from build123d import *

# Parameters (mm, degrees)
SKETCH1_R                  = 10
BOSS_EXTRUDE1_DEPTH        = 30
SKETCH2_R                  = 5.005
CUT_EXTRUDE1_DEPTH         = 20
CUT_EXTRUDE2_DEPTH         = 10
SKETCH4_R                  = 8
CUT_EXTRUDE3_DEPTH         = 4.01
M2X0_4_TAPPED_HOLE1_REACH  = 39.417
M2X0_4_TAPPED_HOLE1_BORE_R = 0.8
M2X0_4_TAPPED_HOLE2_D      = 1.6
M2X0_4_TAPPED_HOLE3_D      = 1.6
M2X0_4_TAPPED_HOLE4_REACH  = 39.417
M2X0_4_TAPPED_HOLE4_BORE_R = 0.8


with BuildPart() as part:
    # Sketch1 → Boss-Extrude1 (new body)
    with BuildSketch(Plane(origin=(0, 0, 0), x_dir=(0, 0, -1), z_dir=(1, 0, 0))):
        Circle(SKETCH1_R)
    extrude(amount=BOSS_EXTRUDE1_DEPTH)

    # Sketch2 → Cut-Extrude1 (cut)
    with BuildSketch(Plane.ZY):
        Circle(SKETCH2_R)
    extrude(amount=-CUT_EXTRUDE1_DEPTH, mode=Mode.SUBTRACT)

    # Sketch3 → Cut-Extrude2 (cut)
    with BuildSketch(Plane(origin=(30, 0, 0), x_dir=(0, 0, -1), z_dir=(1, 0, 0))):
        with BuildLine():
            Line((-6, 0), (-6, 8))
            ThreePointArc((-6, 8), (0, 10), (6, 8))
            Line((6, 8), (6, 0))
            ThreePointArc((6, 0), (0, -6), (-6, 0))
        make_face()
    extrude(amount=-CUT_EXTRUDE2_DEPTH, mode=Mode.SUBTRACT)

    # Sketch4 → Cut-Extrude3 (cut)
    with BuildSketch(Plane(origin=(20, 0, 0), x_dir=(0, 0, -1), z_dir=(1, 0, 0))):
        Circle(SKETCH4_R)
    extrude(amount=CUT_EXTRUDE3_DEPTH, mode=Mode.SUBTRACT)

    # M2x0.4 Tapped Hole1 bore → M2x0.4 Tapped Hole1 (cut, up to next)
    with BuildSketch(Plane(origin=(0, 0, -10), x_dir=(1, 0, 0), z_dir=(0, 0, -1)), mode=Mode.PRIVATE) as m2x0_4_tapped_hole1_sk1:
        with Locations((22.2, 0)):
            Circle(M2X0_4_TAPPED_HOLE1_BORE_R)
    m2x0_4_tapped_hole1_tool1 = extrude(m2x0_4_tapped_hole1_sk1.sketch, amount=-M2X0_4_TAPPED_HOLE1_REACH, mode=Mode.PRIVATE) & part.part
    add(m2x0_4_tapped_hole1_tool1.solids().sort_by_distance((22.2, 0, -10))[0], mode=Mode.SUBTRACT)

    # M2x0.4 Tapped Hole2 (through all)
    with Locations(Plane.XY.offset(10)):
        with Locations((22.2, 0)):
            Hole(M2X0_4_TAPPED_HOLE2_D / 2)

    # M2x0.4 Tapped Hole3 (through all)
    with Locations(Plane.XZ.offset(10)):
        with Locations((22.2, 0)):
            Hole(M2X0_4_TAPPED_HOLE3_D / 2)

    # M2x0.4 Tapped Hole4 bore → M2x0.4 Tapped Hole4 (cut, up to next)
    with BuildSketch(Plane(origin=(0, 10, 0), x_dir=(1, 0, 0), z_dir=(0, 1, 0)), mode=Mode.PRIVATE) as m2x0_4_tapped_hole4_sk1:
        with Locations((3, 0)):
            Circle(M2X0_4_TAPPED_HOLE4_BORE_R)
    m2x0_4_tapped_hole4_tool1 = extrude(m2x0_4_tapped_hole4_sk1.sketch, amount=-M2X0_4_TAPPED_HOLE4_REACH, mode=Mode.PRIVATE) & part.part
    add(m2x0_4_tapped_hole4_tool1.solids().sort_by_distance((3, 10, 0))[0], mode=Mode.SUBTRACT)


solid = part.part
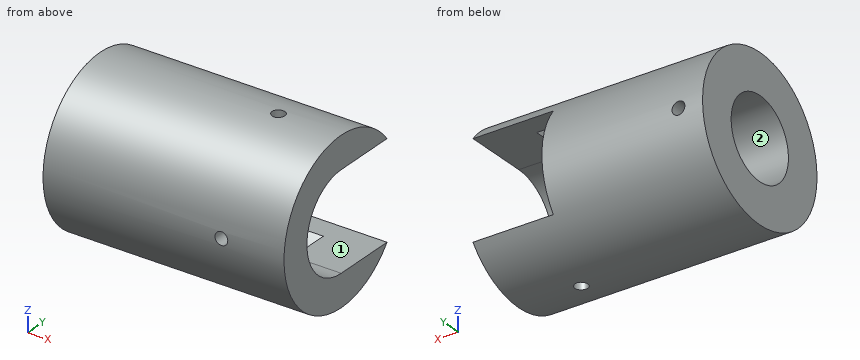
Work out the finished part from the listing and answer in its coordinate system (mm). Face numbers are marked on the shaded views. A direction names the side the tool comes from. Coordinates: 2 decimals unless noted, no trailing zeros. Order: outer loops, then holes, each group sorted by start corner. A loop starts at its lowest first (then second) coordinate and runs counter-clockwise, first axis right, second up. Notation, with made-up numbers: (-27, -34.75) - (-13, -34.75) arc R26 cw to (-13, 1.25) - close; hole circle Ø1 at (60, -16.75). An arc over 180 degrees is marked (long way). Put each result on its own line as item: value. Start each with the question number.
1) For the marked faces 1 and 2, determine the directions among +Z, -Z, +X, -X, +Y, -Y from which every point of the face is accessible in a straight line to the end or side of a thin tool.
2) Find section A-A (z = 0). Give the vertices of the cut face in (x, y) (3 decimals).
3) Flat-ended cylindrical pins translate along their axes: pin 1 (6.5 mm diameter, centred on y = -0.5, z = -3.5, fed in from -X); pin 2 (3 mm diameter, centred on x = 21, y = -5.5, fed in from -Z); pin 3 (4 mm diameter, centred on x = 26.5, y = 5.5, fed in from -Z); pin 4 (2 mm diameter, centred on x = 21, y = -7, fed in from -Z). Find the tip coordinate at first contact, or state that the pin passes through.
4) Find section D-D (z = 7.25). Give the vertices of the cut face in (x, y).
5) Find section B-B (x = 22.2). Give the vertices of the cut face in (y, z), plus the area to 3 significant figures.
6) Find section C-C (y = 4.5). Give the vertices of the cut face in (x, z), plus the area to 3 significant figures.
7) Find the intervals of material crossed by line 1 (X direction, y = 7.6, z = 0); line 2 (X direction, y = -0.75, z = -7.25); line 3 (Z direction, x = 11, y = 0.25), in increasing order. Write a range as from..to.
Results list:
1. face 1: +X, +Y
1. face 2: +X, -X
2. outline: (0, -10) - (21.4, -10) - (21.4, -8) - (20, -8) - (20, -5.005) - (0, -5.005) - close; (0, 5.005) - (2.2, 5.005) - (2.2, 10) - (0, 10) - close; (3.8, 5.005) - (20, 5.005) - (20, 10) - (3.8, 10) - close; (23, -10) - (30, -10) - (30, -6) - (24.01, -6) - (24.01, -8) - (23, -8) - close
3. pin 1: stops at x = 0
3. pin 2: stops at z = -9.17
3. pin 3: stops at z = -9.37
3. pin 4: stops at z = -8
4. outline: (0, -6.89) - (30, -6.89) - (30, 6.89) - (0, 6.89) - close; hole (20, -3.38) - (24.01, -3.38) - (24.01, 3.38) - (20, 3.38) - close
5. outline: (-9.97, -0.8) arc R10 ccw to (-0.8, -9.97) - (-0.8, -7.96) arc R8 cw to (-7.96, -0.8) - close; (-9.97, 0.8) - (-7.96, 0.8) arc R8 cw to (-0.8, 7.96) - (-0.8, 9.97) arc R10 ccw to start; (0.8, -9.97) arc R10 ccw to (8, -6) - (5.29, -6) arc R8 cw to (0.8, -7.96) - close; (0.8, 7.96) arc R8 cw to (5.29, 6) - (8, 6) arc R10 ccw to (0.8, 9.97) - close
5. area: 77.2 mm^2
6. outline: (0, -8.93) - (30, -8.93) - (30, -6) - (24.01, -6) - (24.01, -6.61) - (20, -6.61) - (20, -2.19) - (0, -2.19) - close; (0, 2.19) - (20, 2.19) - (20, 6.61) - (24.01, 6.61) - (24.01, 6) - (30, 6) - (30, 8.93) - (0, 8.93) - close
6. area: 323 mm^2
7. line 1: x = 0..2.2, 3.8..20
7. line 2: x = 0..20, 24.01..30
7. line 3: z = -10..-5, 5..10
